Could you check a few things on this model? Use its own coordinates, in mm. Face numbers are marked on the shaded views. A direction names the side the tool comes from. Give positions to 0.01 mm unless a question says otherwise; leave off trailing zeros. Order: outer loops, then holes, each group sorted by start corner. A loop starts at its lowest first (then second) coordinate and runs counter-clockwise, first axis right, second up. Notation, with made-up numbers: (7.5, 3.25) -> (32.5, 3.25) arc R18 cw to (32.5, 21.25) -> close; hole circle Ø9 at (7, 55). An arc over 180 degrees is marked (long way). Write each question's results on one line, items separated by ' | '.
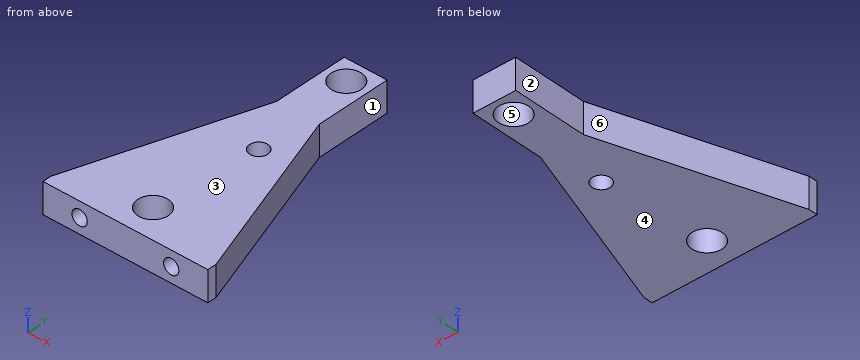
```python
from build123d import *

# Parameters (mm, degrees)
ESQUISSE1_W             = 7
ESQUISSE1_H             = 42
BOSS_EXTRU_1_DEPTH      = 5
ESQUISSE2_R             = 2.5
ENL_V_MAT_EXTRU_1_DEPTH = 43.87190222
ESQUISSE3_R             = 1.5
ENL_V_MAT_EXTRU_2_DEPTH = 10
BOSS_EXTRU_2_DEPTH      = 5
ESQUISSE7_W             = 27
ESQUISSE7_H             = 5
BOSS_EXTRU_3_DEPTH      = 1.49
TROU_TARAUD_M32_D       = 2.5
TROU_TARAUD_M32_DEPTH   = 8.5
TROU_TARAUD_M32_TIP     = 0.751075774


with BuildPart() as part:
    # Esquisse1 → Boss.-Extru.1 (new body)
    with BuildSketch(Plane.XY):
        with Locations((3.5, 21)):
            Rectangle(ESQUISSE1_W, ESQUISSE1_H)
    extrude(amount=BOSS_EXTRU_1_DEPTH)

    # Esquisse2 → Enlèv. mat.-Extru.1 (cut, through all)
    with BuildSketch(Plane(origin=(0, 0, 0), x_dir=(-1, 0, 0), z_dir=(0, 0, -1))):
        with Locations((-3.5, 38.5)):
            Circle(ESQUISSE2_R)
        with Locations((-3.5, 3.5)):
            Circle(ESQUISSE2_R)
    extrude(amount=-ENL_V_MAT_EXTRU_1_DEPTH, mode=Mode.SUBTRACT)

    # Esquisse3 → Enlèv. mat.-Extru.2 (cut)
    with BuildSketch(Plane(origin=(0, 0, 0), x_dir=(-1, 0, 0), z_dir=(0, 0, -1))):
        with Locations((-5, 21)):
            Circle(ESQUISSE3_R)
    extrude(amount=-ENL_V_MAT_EXTRU_2_DEPTH, mode=Mode.SUBTRACT)

    # Esquisse4 → Boss.-Extru.2 (add)
    with BuildSketch(Plane(origin=(0, 0, 0), x_dir=(-1, 0, 0), z_dir=(0, 0, -1))):
        Polygon((-7, 29.75), (-17, 0), (-7, 0), align=None)
        Polygon((10, 0), (0, 0), (0, 29.75), align=None)
    extrude(amount=-BOSS_EXTRU_2_DEPTH)

    # Esquisse7 → Boss.-Extru.3 (add)
    with BuildSketch(Plane(origin=(0, 0, 0), x_dir=(-1, 0, 0), z_dir=(0, -1, 0))):
        with Locations((-3.5, -2.5)):
            Rectangle(ESQUISSE7_W, ESQUISSE7_H)
    extrude(amount=BOSS_EXTRU_3_DEPTH)

    # Trou taraudé M32
    with Locations(Plane(origin=(0, -1.49, 0), x_dir=(-1, 0, 0), z_dir=(0, -1, 0))):
        with Locations((4, -2.5), (-11, -2.5)):
            Hole(TROU_TARAUD_M32_D / 2, depth=TROU_TARAUD_M32_DEPTH)
            with Locations((0, 0, -(TROU_TARAUD_M32_DEPTH + TROU_TARAUD_M32_TIP / 2))):  # 118° drill point
                Cone(0, TROU_TARAUD_M32_D / 2, TROU_TARAUD_M32_TIP, mode=Mode.SUBTRACT)


solid = part.part
```
Q1. Suppose I cut it at C-C on y = 21. Please give me the cut outline in (x, z).
Here are the results:
outline: (-2.94, 0) -> (3.5, 0) -> (3.5, 5) -> (-2.94, 5) -> close; (6.5, 0) -> (9.94, 0) -> (9.94, 5) -> (6.5, 5) -> close
Q2. Suppose I cut it at D-D on x = -0.5. Please give me the cut outline in (y, z).
Here are the results:
outline: (-1.49, 0) -> (28.26, 0) -> (28.26, 5) -> (-1.49, 5) -> close
Q3. Suppose I cut it at B-B on x = 5. Please give me the cut outline in (y, z).
Here are the results:
outline: (-1.49, 0) -> (1.5, 0) -> (1.5, 5) -> (-1.49, 5) -> close; (5.5, 0) -> (19.5, 0) -> (19.5, 5) -> (5.5, 5) -> close; (22.5, 0) -> (36.5, 0) -> (36.5, 5) -> (22.5, 5) -> close; (40.5, 0) -> (42, 0) -> (42, 5) -> (40.5, 5) -> close
Q4. For the marked faces 1, 2 and 3, which set-ups out of +Z, -Z, +X, -X, +Y, -Y let a thin tool reach every point of the face, with its end or its side?
Here are the results:
face 1: +Z, -Z, +X, +Y | face 2: +Z, -Z, -X, +Y | face 3: +Z, +X, -X, +Y, -Y
Q5. I'm going to push flat-ended pins straight in: pin 1 Ø1 at (x, y) = (-4, 18.5) entering from +Z; pin 2 Ø4 at (x, y) = (3.5, 3.5) entering from +Z; pin 3 Ø1.5 at (y, z) = (36.5, 3.5) entering from -X; pin 4 Ø2 at (x, z) = (11, 2.5) entering from -Y. Where does each tip first touch, or does it pass through?
Here are the results:
pin 1: stops at z = 5 | pin 2: passes through | pin 3: stops at x = 0 | pin 4: stops at y = 7.16
Q6. Thinking about a two-plate mould opening in Y: for the marked faces 4, 5 and 6, which applies, +Y half, -Y half, draft (parallel to the pull), parting line (faces both ways), or undercut?
Here are the results:
face 4: draft | face 5: undercut | face 6: +Y half
Q7. Suppose I cut it at A-A on y = 38.5. Please give me the cut outline in (x, z), and give its area (3 significant figures).
Here are the results:
outline: (0, 0) -> (1, 0) -> (1, 5) -> (0, 5) -> close; (6, 0) -> (7, 0) -> (7, 5) -> (6, 5) -> close | area: 10.0 mm²
Q8. I need wall thicknesses on line 1 along Z through (x, y) = (11, 1.25); line 2 along X through (y, z) = (0.5, 2.85); line 3 along X through (y, z) = (33, 4). Which ranges of each line are inside material? Lowest first, please.
Here are the results:
line 1: z = 0 to 1.25, 3.75 to 5 | line 2: x = -9.83 to -5.2, -2.8 to 9.8, 12.2 to 16.83 | line 3: x = 0 to 7
